Job drawing, mm, ordinate dimensions from the low corner. One solid piece. A direction names the side the tool comes from. Give positions to 0.01 mm unless a question says otherwise; leave off trailing zeros. Loops run counter-clockwise (first coordinate to the right, second up) from the corner with the lowest first, then second, coordinate; pieces in that order, holes last. Notation, with made-up numbers: (85, -15) -> (89, -15) arc R15 cw to (89, -8) -> close; hole circle Ø9 at (-3, 58.5). An arc over 180 degrees is marked (long way). Use one line per item in the form item = value.
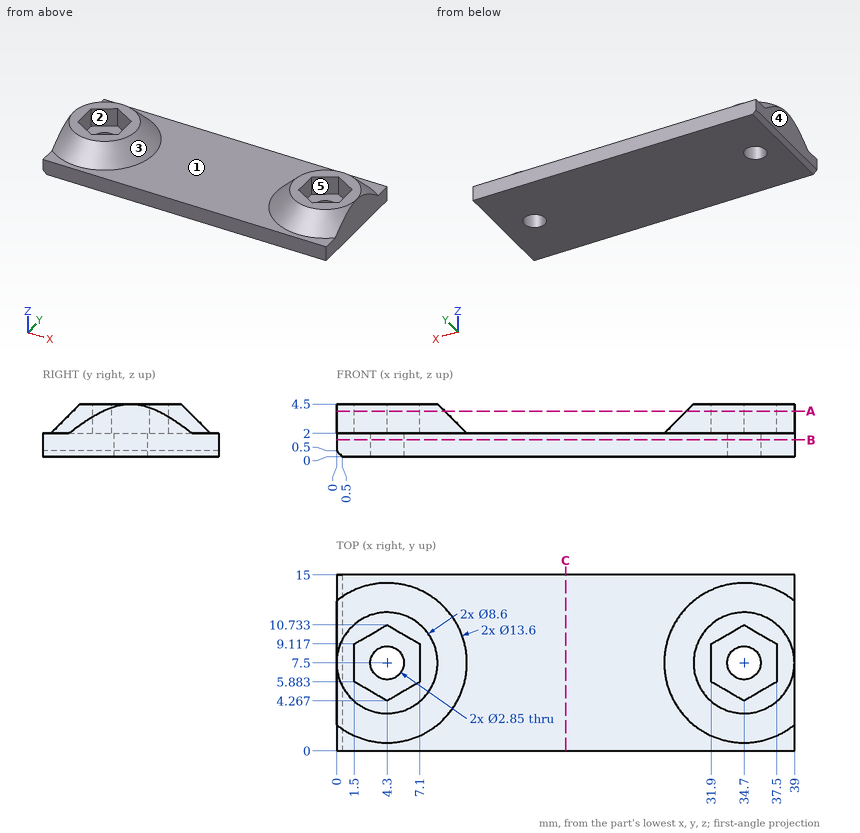
1. Cut at C-C, the plane x = 19.5. Write the cut outline in (y, z).
Result sheet:
outline = (0, 0) -> (15, 0) -> (15, 2) -> (0, 2) -> close
2. Cut at B-B, the plane z = 1.45. State how many separate pieces and enclosed holes the cut face has, then the cut area to 3 significant figures.
Result sheet:
separate_pieces = 1
enclosed_holes = 2
area = 572 mm^2
3. Tool access for the marked faces 4 and 5: list every direction of +Z, -Z, +X, -X, +Y, -Y with a clear straight run to the whole face (end or side of a thin tool).
Result sheet:
face_4 = +Z, -Z, -X, +Y, -Y
face_5 = +Z
4. Drill centre lines: line 1 (Y direction, x = 34.7, z = 0.9) (1 decimal); line 2 (X direction, y = 7.75, z = 3.3) (1 decimal); line 3 (X direction, y = 4.75, z = 4.2) (1 decimal). Where is each one in solid material? Low to high.
Result sheet:
line_1 = 0 to 6.1, 8.9 to 15
line_2 = 0 to 1.5, 7.1 to 9.8, 29.2 to 31.9, 37.5 to 39
line_3 = 0.6 to 3.5, 5.1 to 8, 31 to 33.9, 35.5 to 38.4
5. Mould opens along Y. For the marked faces 1, 2 and 3 say: pulls with the +Y half, pulls with the -Y half, needs draft (parallel to the pull), parting line crosses it, or undercut.
Result sheet:
face_1 = needs draft
face_2 = undercut
face_3 = parting line crosses it
6. Drop a flat-ended pin along its axis: P1, Ø2.5, axis at x = 4.3, y = 7.5, coming from the +Z side. Give the stop position or say it passes through.
Result sheet:
P1 = through
7. Cut at A-A, the plane z = 3.9. Write the cut outline in (x, y).
Result sheet:
outline = (0, 5.15) arc R4.9 ccw (long way) to (0, 9.85) -> close; (39, 5.15) -> (39, 9.85) arc R4.9 ccw (long way) to start; hole (1.5, 5.88) -> (4.3, 4.27) -> (7.1, 5.88) -> (7.1, 9.12) -> (4.3, 10.73) -> (1.5, 9.12) -> close; hole (31.9, 5.88) -> (34.7, 4.27) -> (37.5, 5.88) -> (37.5, 9.12) -> (34.7, 10.73) -> (31.9, 9.12) -> close
